Design review of the part built by this model. Coordinates are the model's own, in mm. Face numbers are marked on the shaded views. A direction names the side the tool comes from. Round coordinates to 2 decimals unless told otherwise and drop trailing zeros. Order: outer loops, then holes, each group sorted by start corner. A loop starts at its lowest first (then second) coordinate and runs counter-clockwise, first axis right, second up.
from build123d import *

# Parameters (mm, degrees)
SKETCH1_W                   = 260.35
SKETCH1_H                   = 158.75
BOSS_EXTRUDE1_DEPTH         = 25.4
SHELL1_T                    = -3.175
SKETCH2_W                   = 50.8
SKETCH2_H                   = 50.8
BOSS_EXTRUDE2_DEPTH         = 184.15
SHELL2_START                = -161.925
SHELL2_OUTLINE_W            = 44.45
SHELL2_OUTLINE_H            = 44.45
SHELL2_DEPTH                = 184.15
BOSS_EXTRUDE3_DEPTH         = 3.175
FILLET1_R                   = 2.54
SKETCH6_W                   = 31.75
SKETCH6_H                   = 25.4
SKETCH6_R                   = 4.7625
BOSS_EXTRUDE4_DEPTH         = 6.35
FILLET2_R                   = 5.08
SKETCH7_W                   = 25.4
SKETCH7_H                   = 25.4
SKETCH7_R                   = 4.7625
BOSS_EXTRUDE5_DEPTH         = 6.35
FILLET3_R                   = 5.08
FILLET3_OF_MIRROR3_R        = 5.08
F_1_4_0_25_DIAMETER_HOLE1_D = 6.35


# Read off the part's stored shape, not the designer's step: Shell2
with BuildPart() as part:
    # Sketch1 → Boss-Extrude1 (new body)
    with BuildSketch(Plane(origin=(0, 0, 0), x_dir=(1, 0, 0), z_dir=(0, 1, 0))):
        Rectangle(SKETCH1_W, SKETCH1_H)
    extrude(amount=BOSS_EXTRUDE1_DEPTH)

    # Shell1
    shell1_openings = [part.faces().sort_by_distance(p)[0] for p in [
        (0, 0, 0),
    ]]
    offset(amount=SHELL1_T, openings=shell1_openings, kind=Kind.INTERSECTION)

    # Sketch2 → Boss-Extrude2 (add)
    with BuildSketch(Plane.XZ.offset(-22.225)):
        Rectangle(SKETCH2_W, SKETCH2_H)
    extrude(amount=BOSS_EXTRUDE2_DEPTH)

    # Shell2 outline → Shell2 (cut)
    with BuildSketch(Plane(origin=(0, 0, 0), x_dir=(1, 0, 0), z_dir=(0, 1, 0)).offset(SHELL2_START)):
        Rectangle(SHELL2_OUTLINE_W, SHELL2_OUTLINE_H)
    extrude(amount=SHELL2_DEPTH, mode=Mode.SUBTRACT)

    # Sketch4 → Boss-Extrude3 (add, symmetric)
    with BuildSketch(Plane.XY):
        Polygon((25.4, -9.525), (63.5, 22.225), (123.01410253, 22.225), (25.4, -59.120085442), align=None)
    boss_extrude3 = extrude(amount=BOSS_EXTRUDE3_DEPTH, both=True)

    # Mirror1: Boss-Extrude3 across plane
    add(boss_extrude3.mirror(Plane(origin=(0, 0, 0), x_dir=(0, 0, 1), z_dir=(1, 0, 0))))

    # Fillet1
    fillet1_edges = [part.edges().sort_by_distance(p)[0] for p in [
        (-130.175, 25.4, 0),
        (0, 25.4, 79.375),
        (130.175, 25.4, 0),
        (0, 25.4, -79.375),
    ]]
    fillet(fillet1_edges, radius=FILLET1_R)

    # Sketch6 → Boss-Extrude4 (add)
    with BuildSketch(Plane.XY.offset(14.2875)):
        with Locations((41.275, -149.225)):
            Rectangle(SKETCH6_W, SKETCH6_H)
        with Locations((44.45, -149.225)):
            Circle(SKETCH6_R, mode=Mode.SUBTRACT)
    boss_extrude4 = extrude(amount=-BOSS_EXTRUDE4_DEPTH)

    # Mirror2: Boss-Extrude4 across plane
    add(boss_extrude4.mirror(Plane.XY))

    # Fillet2
    fillet2_edges = [part.edges().sort_by_distance(p)[0] for p in [
        (57.15, -161.925, -11.1125),
        (57.15, -136.525, -11.1125),
        (57.15, -136.525, 11.1125),
        (57.15, -161.925, 11.1125),
    ]]
    fillet(fillet2_edges, radius=FILLET2_R)

    # Sketch7 → Boss-Extrude5 (add)
    with BuildSketch(Plane(origin=(0, 0, 0), x_dir=(0, 0, -1), z_dir=(1, 0, 0))):
        with Locations((-38.1, -144.4625)):
            Rectangle(SKETCH7_W, SKETCH7_H)
        with Locations((-38.1, -144.4625)):
            Circle(SKETCH7_R, mode=Mode.SUBTRACT)
    boss_extrude5 = extrude(amount=-BOSS_EXTRUDE5_DEPTH)

    # Fillet3
    fillet3_edges = [part.edges().sort_by_distance(p)[0] for p in [
        (-3.175, -157.1625, 50.8),
        (-3.175, -131.7625, 50.8),
    ]]
    fillet(fillet3_edges, radius=FILLET3_R)

    # Mirror3: Boss-Extrude5 across plane
    add(boss_extrude5.mirror(Plane.XY))

    # Fillet3 of Mirror3
    fillet3_of_mirror3_edges = [part.edges().sort_by_distance(p)[0] for p in [
        (-3.175, -157.1625, -50.8),
        (-3.175, -131.7625, -50.8),
    ]]
    fillet(fillet3_of_mirror3_edges, radius=FILLET3_OF_MIRROR3_R)

    # 1/4 (0.25) Diameter Hole1 (through all)
    with Locations(Plane(origin=(0, 25.4, 0), x_dir=(1, 0, 0), z_dir=(0, 1, 0))):
        with Locations((-104.775, 53.975), (-34.925, 53.975), (34.925, 53.975), (104.775, 53.975)):
            f_1_4_0_25_diameter_hole1 = Hole(F_1_4_0_25_DIAMETER_HOLE1_D / 2)

    # Mirror4: 1/4 (0.25) Diameter Hole1 across plane
    add(f_1_4_0_25_diameter_hole1.mirror(Plane.XY), mode=Mode.SUBTRACT)


solid = part.part
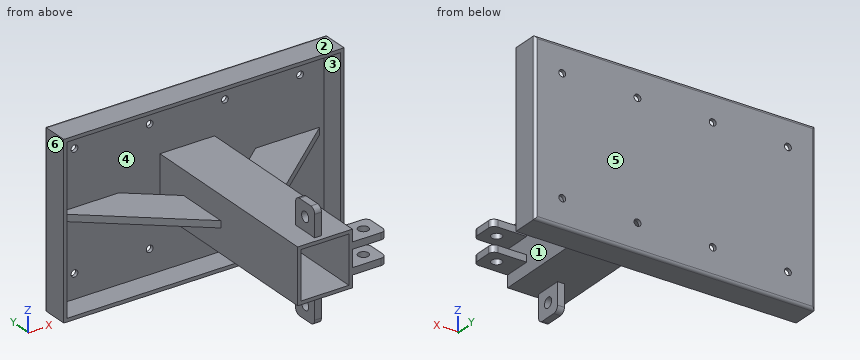
1) To check wall thickness, follow line 1 along Z through (x, y) = (-79.5, 1) (3 decimals); line 2 along Y through (x, z) = (44.45, 12.75) (1 decimal); line 3 along Y through (x, z) = (-4.5, 38.1) (1 decimal). State the ranges of each line that lie inside material, in increasing order.
Results:
line 1: z = -79.375 to -76.2, -3.175 to 3.175, 76.2 to 79.375
line 2: y = -161.9 to -154, -144.5 to -136.5, 22.2 to 25.4
line 3: y = -157.2 to -149.2, -139.7 to -131.8, 22.2 to 25.4
2) Take a section at B-B on z = -38.1. State how many separate pieces and enclosed holes the cut face has, plus the area to 3 significant figures.
Results:
separate pieces: 3
enclosed holes: 0
area: 1,070 mm2
3) Clearance check with flat-ended pins moving along their axes: P1, Ø10, axis at x = -104.775, z = 53.975, coming from the -Y side (3 decimals); P2, Ø15, axis at y = -90, z = -12.5, coming from the -X side; P3, Ø1.5, axis at x = -64, y = -2.5, coming from the +Z side (3 decimals). State where each tip first meets the part, or that it passes through.
Results:
P1: stops at y = 22.225
P2: stops at x = -25.4
P3: stops at z = 3.175
4) Take a section at C-C on x = 5. Give the boundary of the cut face in (y, z) (3 decimals).
Results:
outline: (-161.925, -25.4) - (22.225, -25.4) - (22.225, -76.2) - (0, -76.2) - (0, -79.375) - (22.86, -79.375) arc R2.54 ccw to (25.4, -76.835) - (25.4, 76.835) arc R2.54 ccw to (22.86, 79.375) - (0, 79.375) - (0, 76.2) - (22.225, 76.2) - (22.225, 25.4) - (-161.925, 25.4) - (-161.925, 22.225) - (22.225, 22.225) - (22.225, -22.225) - (-161.925, -22.225) - close
5) The part is to be moulded in two halves that separate along X. For the marked faces 4, 5 and 6, say which applies: released by +X, released by -X, zero draft, split by the parting line, or undercut.
Results:
face 4: undercut
face 5: zero draft
face 6: released by -X
6) For the marked faces 1, 2 and 3, list the 3-axis set-ups (+Z, -Z, +X, -X, +Y, -Y) from which the entire face can be reached by the end or side of a thin tool; tool diameter is ignored.
Results:
face 1: none
face 2: +Z, +X, -X, +Y, -Y
face 3: -Y
7) Take a section at A-A on y = -68.5. Give the boundary of the cut face in (x, z) (3 decimals), plus the area to 3 significant figures.
Results:
outline: (-25.4, -25.4) - (25.4, -25.4) - (25.4, 25.4) - (-25.4, 25.4) - close; hole (-22.225, -22.225) - (22.225, -22.225) - (22.225, 22.225) - (-22.225, 22.225) - close
area: 605 mm2
